Autodesk Inventor part; units mm, degrees
ref_plane "YZ Plane" through (0, 0, 0) normal (1, 0, 0) x (0, 1, 0)
ref_plane "XZ Plane" through (0, 0, 0) normal (0, 1, 0) x (-1, 0, 0)
ref_plane "XY Plane" through (0, 0, 0) normal (0, 0, 1) x (1, 0, 0)
sketch "Эскиз1" plane through (0, 0, 0) normal (0, 0, 1) x (1, 0, 0)
  line L0 (-7, -10) -> (7, -10)
  line L1 (7, -10) -> (7, 10)
  line L2 (7, 10) -> (-7, 10)
  line L3 (-7, 10) -> (-7, -10)
  line L4 (-7, -10) -> (7, 10) construction
  line L5 (7, -10) -> (-7, 10) construction
  point P0 (0, 0)
  dimension "d0" = 14
  dimension "d1" = 20
extrude "Выдавливание1" add sketch "Эскиз1" along normal blind 3
sketch "Эскиз2" plane through (0, 0, 0) normal (0, 0, -1) x (-1, 0, 0)
  line L0 (7, -10) -> (-7, -10)
  line L1 (7, 10) -> (7, -10)
  line L2 (-7, 10) -> (7, 10)
  line L3 (-7, -10) -> (-7, 10)
  line L4 (7, -10) -> (7, -7)
  line L5 (7, 10) -> (7, -10) construction
  line L6 (7, -10) -> (-7, -10)
  line L7 (7, -7) -> (-7, -7)
  line L8 (-7, -7) -> (-7, -10)
  line L9 (-7, -10) -> (7, -10)
  line L10 (7, -10) -> (7, -7)
  point P0 (0, 0)
  dimension "d4" = 3
extrude "Выдавливание2" add sketch "Эскиз2" along normal blind 6 contours L0 L3 L7 L1
sketch "Эскиз3" plane through (-7, -7, 0) normal (0, 1, 0) x (1, 0, 0)
  line L0 (14, 6) -> (0, 6)
  line L1 (14, 0) -> (0, 0)
  line L2 (14, 0) -> (14, 6)
  line L3 (0, 6) -> (14, 6)
  line L4 (0, 0) -> (0, 6)
  line L5 (14, 6) -> (14, 3) construction
  line L6 (14, 0) -> (14, 6) construction
  line L7 (14, 3) -> (0, 3)
  line L8 (0, 3) -> (0, 6)
  line L9 (0, 6) -> (14, 6)
  line L10 (14, 6) -> (14, 3)
  point P0 (7, 0)
  dimension "d7" = 3
extrude "Выдавливание3" add sketch "Эскиз3" along normal blind 6 contours L2 L7 L4 L0
sketch "Эскиз4" plane through (0, 0, -6) normal (0, 0, -1) x (-1, 0, 0)
  line L0 (-7, -10) -> (7, -10)
  line L1 (7, -10) -> (7, -1)
  line L2 (-7, -1) -> (7, -1)
  line L3 (-7, -10) -> (-7, -1)
  line L4 (-7, -1) -> (7, -1) construction
  line L5 (-7, -1) -> (-7, -4) construction
  line L6 (-7, -4) -> (7, -4)
  line L7 (7, -4) -> (7, -1)
  line L8 (7, -1) -> (-7, -1)
  line L9 (-7, -1) -> (-7, -4)
  point P0 (0, 0)
  dimension "d10" = 3
extrude "Выдавливание4" add sketch "Эскиз4" along normal blind 28 contours L3 L2 L1 L6
sketch "Эскиз6" plane through (0, 0, 3) normal (0, 0, 1) x (1, 0, 0)
  line L0 (-7, -10) -> (7, -10)
  line L1 (7, -10) -> (7, 10)
  line L2 (7, 10) -> (-7, 10)
  line L3 (-7, 0) -> (7, 0) construction
  line L4 (7, -7) -> (7, 10) construction
  line L5 (7, 10) -> (-7, 10) construction
  line L6 (0, 10) -> (0, -10) construction
  line L7 (0, 0) -> (0, 10) construction
  line L8 (0, 5) -> (-7, 5) construction
  line L9 (-7, 10) -> (-7, -10) construction
  line L10 (0, 5) -> (7, 5) construction
  line L11 (0, -10) -> (0, 0) construction
  line L12 (0, -5) -> (7, -5) construction
  circle A0 centre (0, 5) radius 2
  circle A1 centre (0, -5) radius 2
  line L13 (-7, 10) -> (-7, -10)
  point P0 (-5.8649, 10)
  dimension "d15" = 4
  dimension "d16" = 4
extrude "Выдавливание6" cut sketch "Эскиз6" against normal up to surface (6 mm away) contours A0 | A1
sketch "Эскиз7" plane through (-7, -10, 3) normal (0, -1, 0) x (1, 0, 0)
  line L0 (14, -9) -> (14, 0)
  line L1 (0, 0) -> (14, 0)
  line L2 (0, 0) -> (0, -9)
  line L3 (14, -9) -> (0, -9)
  line L4 (0, -9) -> (14, -9)
  line L5 (0, -9) -> (0, -37)
  line L6 (14, -37) -> (0, -37)
  line L7 (14, -9) -> (14, -37)
  line L8 (0, 0) -> (14, 0)
  line L9 (0, -6) -> (0, -37)
  line L10 (14, 0) -> (0, -37)
  line L11 (0, -37) -> (14, -37)
  line L12 (14, -9) -> (14, 0)
  line L13 (14, 0) -> (14, -37)
  point P0 (7, -3)
extrude "Выдавливание7" cut sketch "Эскиз7" against normal blind 28 contours L3 L10 L0 | L7 L6 L10 L3
properties part number "Side control"
Build history of the part. All positions in model axes, mm. A direction names the side the tool comes from. Round coordinates to 2 decimals unless told otherwise and drop trailing zeros. Write each loop counter-clockwise with the first axis right and the second up, starting at its lowest first coordinate (ties: lowest second). Pieces come first, ordered by that corner, then holes.
1) Pin check, flat tips, straight feed: pin 1 (6 mm diameter, centred on y = -4.5, z = -29, fed in from +X); pin 2 (6 mm diameter, centred on x = -2.5, z = -19, fed in from +Y); pin 3 (3 mm diameter, centred on x = -2, y = -6.5, fed in from -Z); pin 4 (2 mm diameter, centred on y = 5, z = -2.5, fed in from +X). Stop position of each tip, or through.
2) Band-saw the part on B-B, the plane y = -5. List the corners of the cut face in (x, z), and give its area (3 significant figures).
3) Drill centre lines: probe 1 along Y at (x, z) = (0, 1.2); probe 2 along Z at (x, y) = (2, 4.5); probe 3 along Y at (x, z) = (-5.75, -5.5). Where is each one in solid material? Low to high.
4) Band-saw the part on D-D, the plane y = 0.25. List the corners of the cut face in (x, z), and give its area (3 significant figures).
5) Band-saw the part on C-C, the plane x = 5.5. List the corners of the cut face in (y, z).
6) Mould opens along Z. For faces 5 (the flat face through (-1, 2, 0)), 6 (the flat face through (-7, -2, -10)), 7 (the flat face through (-1, -4, -3)), 8 (the flat face through (0, 0, 3)) say: +Z half, -Z half, draft (parallel to the pull), parting line (faces both ways), or undercut.
7) 3-axis set-ups, long thin cutter, end or side, ignore diameter. For faces 1 (the flat face through (-2, -7, -6)), 2 (the flat face through (-1, -7, -1)), 3 (the flat face through (-4, -1, -11)), 4 (the cylindrical face through (0, -7, 2)): which of +Z, -Z, +X, -X, +Y, -Y reach the whole face in a straight line?
8) Band-saw the part on A-A, the plane y = -2. List the corners of the cut face in (x, z).
Ans:
1. pin 1: stops at x = -3.99
1. pin 2: stops at y = -1
1. pin 3: stops at z = -6
1. pin 4: passes through
2. outline: (-7, -6) - (3.59, -6) - (4.73, -3) - (-7, -3) - close; (-7, 0) - (-2, 0) - (-2, 3) - (-7, 3) - close; (2, 0) - (5.86, 0) - (7, 3) - (2, 3) - close
2. area: 61.8 mm2
3. probe 1: y = -10 to -7, -3 to 3, 7 to 10
3. probe 2: z = 0 to 3
3. probe 3: y = -10 to -1
4. outline: (-7, 0) - (5.86, 0) - (7, 3) - (-7, 3) - close
4. area: 40.3 mm2
5. outline: (-10, -0.96) - (-7, -0.96) - (-7, 0) - (10, 0) - (10, 3) - (-10, 3) - close
6. face 5: undercut
6. face 6: draft
6. face 7: undercut
6. face 8: +Z half
7. face 1: -Z, +X, -X, -Y
7. face 2: +X, -X, +Y
7. face 3: -Z, +X, -X, +Y
7. face 4: +Z
8. outline: (-7, -34) - (4.73, -3) - (-7, -3) - close; (-7, 0) - (5.86, 0) - (7, 3) - (-7, 3) - close
